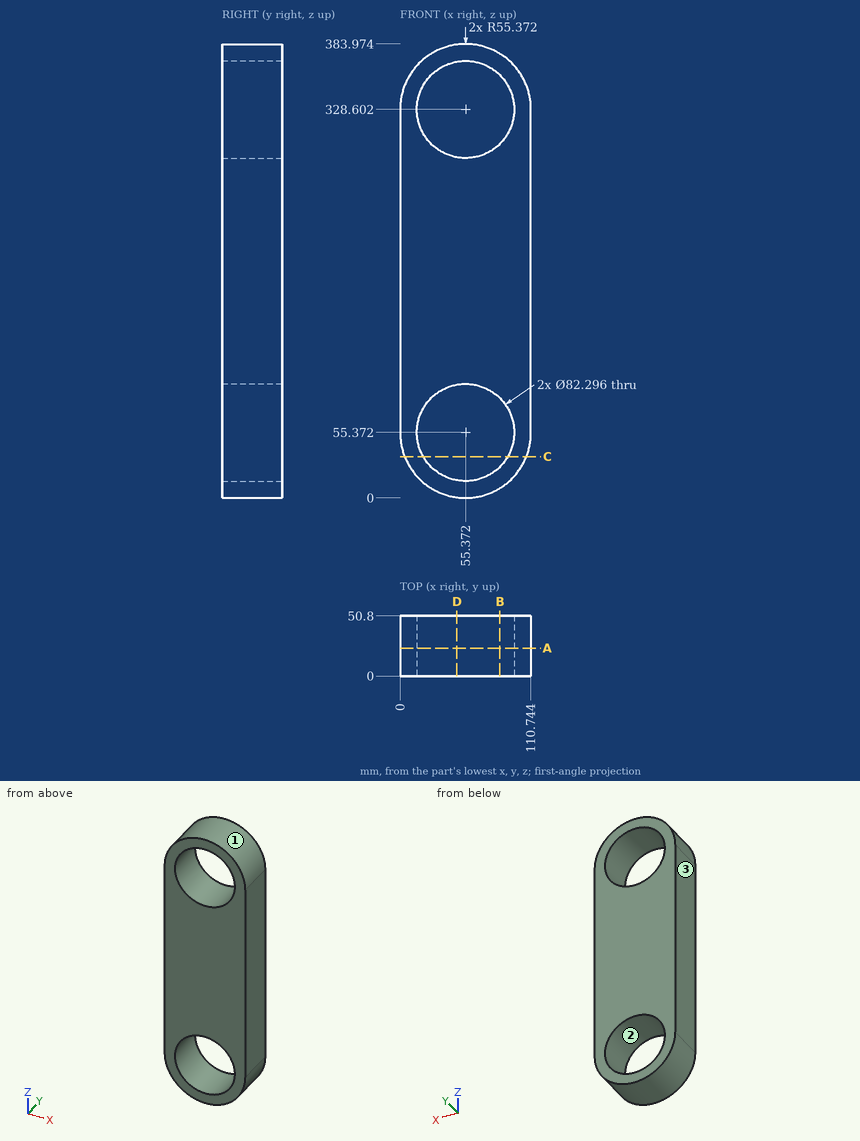
Verification items for this drawing (mm, ordinates from the low corner). Coordinates: 2 decimals unless noted, no trailing zeros. Write each loop counter-clockwise with the first axis right and the second up, starting at its lowest first coordinate (ties: lowest second). Pieces come first, ordered by that corner, then holes. Notation, with made-up numbers: M -37.75,19.5 L -3.75,19.5 A16 cw -3.75,31.5 Z; hole C -26.5,-29 d4. An arc over 180 degrees is marked long. Answer as a JSON object with one key per item and string values.
1. Section check C-C, the plane z = 35. Enter the section's corners in (x, y), plus the area to 3 significant figures.
Answers below:
{"outline": "M 3.88,0 L 19.62,0 L 19.62,50.8 L 3.88,50.8 Z; M 91.12,0 L 106.86,0 L 106.86,50.8 L 91.12,50.8 Z", "area": "1,600 mm²"}
2. Scan lines: L1, parallel to X at y = 47.5, z = 57; L2, parallel to Z at x = 49, y = 45.5; L3, parallel to Z at x = 37, y = 17. Record each from-to range of solid material in increasing order.
Answers below:
{"L1": "x = 0 to 14.26, 96.49 to 110.74", "L2": "z = 0.37 to 14.72, 96.02 to 287.95, 369.25 to 383.61", "L3": "z = 3.14 to 18.55, 92.19 to 291.78, 365.42 to 380.84"}
3. Draft check along Z on the marked faces 1, 2 and 3. Enter one of: released by +Z, released by -Z, zero draft, split by the parting line, or undercut.
Answers below:
{"face 1": "released by +Z", "face 2": "undercut", "face 3": "zero draft"}
4. Section check D-D, the plane x = 48. Enter the section's corners in (y, z), plus the area to 3 significant figures.
Answers below:
{"outline": "M 0,0.49 L 50.8,0.49 L 50.8,14.89 L 0,14.89 Z; M 0,95.85 L 50.8,95.85 L 50.8,288.12 L 0,288.12 Z; M 0,369.08 L 50.8,369.08 L 50.8,383.48 L 0,383.48 Z", "area": "11,200 mm²"}
5. Section check A-A, the plane y = 23.5. Enter the section's corners in (x, z).
Answers below:
{"outline": "M 0,55.37 A55.37 ccw 110.74,55.37 L 110.74,328.6 A55.37 ccw 0,328.6 Z; hole C 55.37,55.37 d82.3; hole C 55.37,328.6 d82.3"}
6. Go/stop test with flat-tipped pins: pin 1 Ø1.5 at (x, y) = (69, 9.5) entering from +Z; pin 2 Ø6 at (x, y) = (79, 24) entering from -Z; pin 3 Ø1 at (x, y) = (18, 40) entering from +Z. Record where each tip stops, or that it passes through.
Answers below:
{"pin 1": "stops at z = 382.46", "pin 2": "stops at z = 3.99", "pin 3": "stops at z = 369.91"}
7. Section check B-B, the plane x = 84.5. Enter the section's corners in (y, z), plus the area to 3 significant figures.
Answers below:
{"outline": "M 0,8.28 L 50.8,8.28 L 50.8,26.31 L 0,26.31 Z; M 0,84.44 L 50.8,84.44 L 50.8,299.54 L 0,299.54 Z; M 0,357.67 L 50.8,357.67 L 50.8,375.69 L 0,375.69 Z", "area": "12,800 mm²"}
